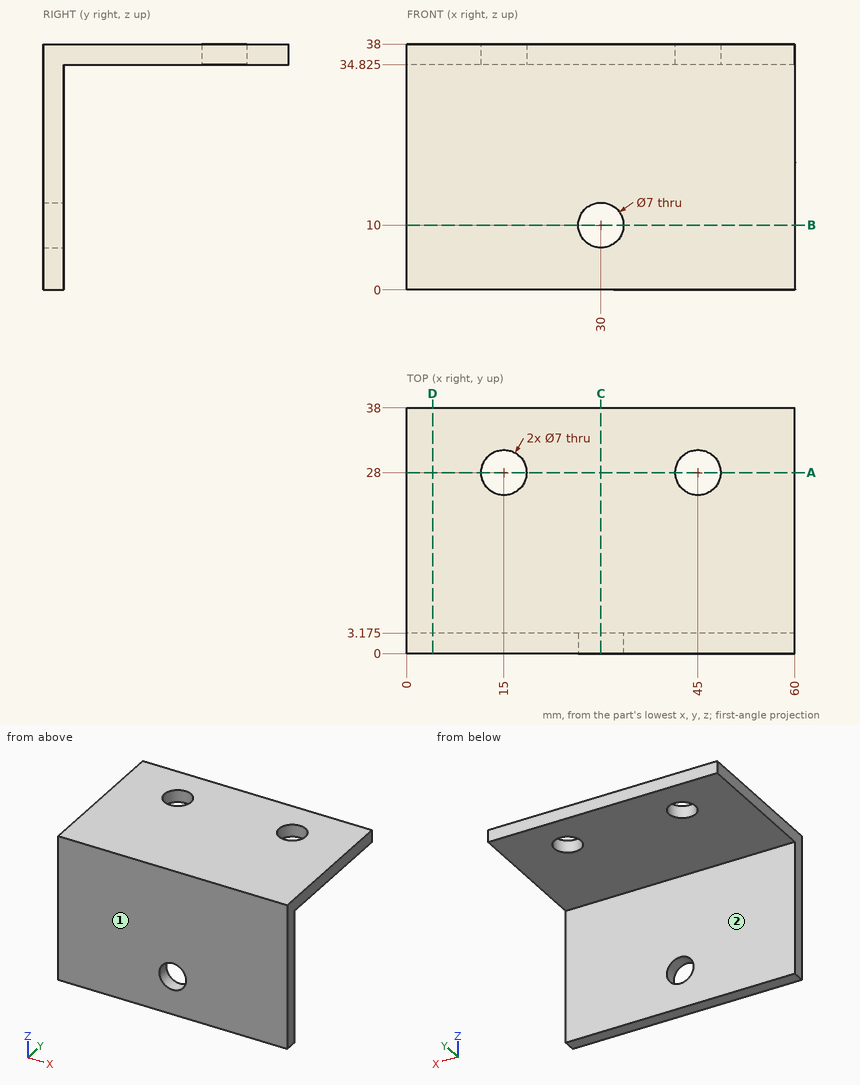
Drawing for the job (mm, zero at the part's lowest x, y, z). A direction names the side the tool comes from. Give positions to 0.01 mm unless a question says otherwise; leave off trailing zeros. Write each loop counter-clockwise with the first axis right and the second up, starting at its lowest first coordinate (ties: lowest second). Pieces come first, ordered by that corner, then holes. Notation, with made-up numbers: M -35,25 L 17,25 A21 cw 17,52 Z; hole C 37.25,23.5 d6. An arc over 180 degrees is marked long. Return JSON: item names as keys, results as strings. Group by question number.
(1) Flat gauge pins, fed straight in: pin 1 Ø17.5 at (x, y) = (35, 18) entering from -Z (3 decimals); pin 2 Ø8 at (x, z) = (40, 17) entering from +Y (3 decimals). Where does each tip first touch, or does it go through?
(2) 3-axis set-ups, long thin cutter, end or side, ignore diameter. For the marked faces 1 and 2: which of +Z, -Z, +X, -X, +Y, -Y reach the whole face in a straight line?
(3) Band-saw the part on D-D (x = 4). Give the cut face in (y, z) (3 decimals), and give its area (3 significant figures).
(4) Band-saw the part on B-B (z = 10). Give the cut face in (x, y) (3 decimals).
(5) Band-saw the part on C-C (x = 30). Give the cut face in (y, z) (3 decimals), and give its area (3 significant figures).
(6) Drill centre lines: L1, parallel to Z at x = 30, y = 2; L2, parallel to Y at x = 15, z = 37.05; L3, parallel to Y at x = 23, z = 31 (3 decimals). Where is each one in solid material? Low to high. Write a range as [from, to].
(7) Band-saw the part on A-A (y = 28). Give the cut face in (x, z) (3 decimals), and give its area (3 significant figures).
Entries:
{
 "1": {"pin 1": "stops at z = 34.825", "pin 2": "stops at y = 3.175"},
 "2": {"face 1": "+Z, -Z, +X, -X, -Y", "face 2": "-Z, +X, -X, +Y"},
 "3": {"outline": "M 0,0 L 3.175,0 L 3.175,34.825 L 38,34.825 L 38,38 L 0,38 Z", "area": "231 mm^2"},
 "4": {"outline": "M 0,0 L 26.5,0 L 26.5,3.175 L 0,3.175 Z; M 33.5,0 L 60,0 L 60,3.175 L 33.5,3.175 Z"},
 "5": {"outline": "M 0,0 L 3.175,0 L 3.175,6.5 L 0,6.5 Z; M 0,13.5 L 3.175,13.5 L 3.175,34.825 L 38,34.825 L 38,38 L 0,38 Z", "area": "209 mm^2"},
 "6": {"L1": "z = [0, 6.5], [13.5, 38]", "L2": "y = [0, 24.5], [31.5, 38]", "L3": "y = [0, 3.175]"},
 "7": {"outline": "M 0,34.825 L 11.5,34.825 L 11.5,38 L 0,38 Z; M 18.5,34.825 L 41.5,34.825 L 41.5,38 L 18.5,38 Z; M 48.5,34.825 L 60,34.825 L 60,38 L 48.5,38 Z", "area": "146 mm^2"}
}
